Verification items for the finished model (mm, model axes). A direction names the side the tool comes from. Coordinates: 2 decimals unless noted, no trailing zeros. Order: outer loops, then holes, each group sorted by start corner. A loop starts at its lowest first (then second) coordinate and runs counter-clockwise, first axis right, second up.
Q1. Cross-section at A-A, the plane z = 10. Record the boundary of the cut face in (x, y), and give its area (3 significant figures).
Q2. Set-up check for faces 1 (the flat face through (-2, -1, 64.15)), 2 (the cylindrical face through (-6.16, 0.14, 1.26)): record each of +Z, -Z, +X, -X, +Y, -Y from which the full face is reachable in a straight line by a thin tool's end or side.
Q3. Depth check by flat-ended pin: P1, Ø10, axis at x = 5.5, z = 22, coming from the +Y side; P2, Ø1, axis at x = -3, y = -7, coming from the -Z side; P3, Ø1.5, axis at x = -3.5, z = 10, coming from the +Y side. Enter the tip coordinate at first touch or a pass-through.
Q4. Draft check along X on faces 3 (the flat face through (-2, -1, 0)), 4 (the flat face through (2, -5, 2.5)), 5 (the cylindrical face through (-6.71, 6.38, 32.51)). Enter one of: pulls with the +X half, pulls with the -X half, needs draft (parallel to the pull), parting line crosses it, or undercut.
Q5. Thickness scan on line 1 (X direction, y = 5, z = 33); line 2 (Z direction, x = 5, y = -5.5); line 3 (Z direction, x = -6, y = 3.5). Record the ranges inside material, lowest first.
from build123d import *


with BuildPart() as part:
    # Sketch1 → Revolve1 (revolve)
    with BuildSketch(Plane.XZ.offset(1.208791209), mode=Mode.PRIVATE) as revolve1_sk:
        with BuildLine():
            Line((6.131868132, 64.15), (-1.868131868, 64.15))
            Line((-1.868131868, 64.15), (-1.868131868, 0))
            Line((-1.868131868, 0), (2.131868132, 0))
            ThreePointArc((2.131868132, 0), (2.485421522, 0.146446609), (2.631868132, 0.5))
            Line((2.631868132, 0.5), (2.631868132, 2))
            ThreePointArc((2.631868132, 2), (2.778314741, 2.353553391), (3.131868132, 2.5))
            Line((3.131868132, 2.5), (4.631868132, 2.5))
            Line((4.631868132, 2.5), (4.631868132, 1.936491673))
            ThreePointArc((4.631868132, 1.936491673), (5.050729302, 0.711746802), (6.131868132, 0))
            ThreePointArc((6.131868132, 0), (6.838974913, 0.292893219), (7.131868132, 1))
            Line((7.131868132, 1), (7.131868132, 63.15))
            ThreePointArc((7.131868132, 63.15), (6.838974913, 63.857106781), (6.131868132, 64.15))
        make_face()
    revolve(revolve1_sk.sketch.rotate(Axis((-1.868131868, -1.208791209, 64.151253994), (0, 0, -1)), 180), axis=Axis((-1.868131868, -1.208791209, 64.151253994), (0, 0, -1)))


solid = part.part
Check values:
1. outline: circle Ø18 at (-1.87, -1.21)
1. area: 254 mm2
2. face 1: +Z, +X, -X, +Y, -Y
2. face 2: -Z
3. P1: stops at y = 7.47
3. P2: stops at z = 2.5
3. P3: stops at y = 7.75
4. face 3: needs draft
4. face 4: undercut
4. face 5: parting line crosses it
5. line 1: x = -8.38 to 4.65
5. line 2: z = 0 to 64.15
5. line 3: z = 2.5 to 64.15
